```python
from build123d import *

# Parameters (mm, degrees)
SKETCH1_W           = 7
SKETCH1_H           = 6
BOSS_EXTRUDE1_DEPTH = 9
CUT_EXTRUDE1_DEPTH  = 2
CUT_EXTRUDE3_DEPTH  = 4
CUT_EXTRUDE4_DEPTH  = 7
SKETCH5_W           = 3
SKETCH5_H           = 2
CUT_EXTRUDE5_DEPTH  = 5
CUT_EXTRUDE8_DEPTH  = 4
CUT_EXTRUDE9_DEPTH  = 4
SKETCH11_W          = 2
SKETCH11_H          = 1
CUT_EXTRUDE12_DEPTH = 4
CUT_EXTRUDE13_DEPTH = 1
SKETCH13_W          = 1
SKETCH13_H          = 1
CUT_EXTRUDE14_DEPTH = 3


with BuildPart() as part:
    # Sketch1 → Boss-Extrude1 (new body)
    with BuildSketch(Plane.XY):
        Rectangle(SKETCH1_W, SKETCH1_H)
    extrude(amount=BOSS_EXTRUDE1_DEPTH)

    # Sketch2 → Cut-Extrude1 (cut)
    with BuildSketch(Plane(origin=(0, 3, 0), x_dir=(1, 0, 0), z_dir=(0, 1, 0))):
        Polygon((3.5, 0), (0.5, 0), (0.5, -3), align=None)
    extrude(amount=-CUT_EXTRUDE1_DEPTH, mode=Mode.SUBTRACT)

    # Sketch3 → Cut-Extrude3 (cut)
    with BuildSketch(Plane(origin=(0, 3, 0), x_dir=(1, 0, 0), z_dir=(0, 1, 0))):
        Polygon((3.5, 0), (0.5, -3), (0.5, -9), (3.5, -9), align=None)
    extrude(amount=-CUT_EXTRUDE3_DEPTH, mode=Mode.SUBTRACT)

    # Sketch4 → Cut-Extrude4 (cut, through all)
    with BuildSketch(Plane(origin=(0, 3, 0), x_dir=(1, 0, 0), z_dir=(0, 1, 0))):
        Polygon((3.5, 0), (1.5, -2), (1.5, -3), (0.5, -5), (0.5, -9), (3.5, -9), align=None)
    extrude(amount=-CUT_EXTRUDE4_DEPTH, mode=Mode.SUBTRACT)

    # Sketch5 → Cut-Extrude5 (cut, through all)
    with BuildSketch(Plane(origin=(0.5, 0, 0), x_dir=(0, 0, -1), z_dir=(1, 0, 0))):
        with Locations((-6.5, -2)):
            Rectangle(SKETCH5_W, SKETCH5_H)
    extrude(amount=-CUT_EXTRUDE5_DEPTH, mode=Mode.SUBTRACT)

    # Sketch7 → Cut-Extrude8 (cut)
    with BuildSketch(Plane(origin=(0, 3, 0), x_dir=(1, 0, 0), z_dir=(0, 1, 0))):
        Polygon((0.5, -3), (-0.5, -4), (-0.5, -9), (0.5, -9), align=None)
    extrude(amount=-CUT_EXTRUDE8_DEPTH, mode=Mode.SUBTRACT)

    # Sketch8 → Cut-Extrude9 (cut, through all)
    with BuildSketch(Plane(origin=(-0.5, 0, 0), x_dir=(0, 0, -1), z_dir=(1, 0, 0))):
        Polygon((-4, 3), (-5, 2), (-5, 1), (-7, 1), (-7, 3), align=None)
    extrude(amount=-CUT_EXTRUDE9_DEPTH, mode=Mode.SUBTRACT)

    # Sketch11 → Cut-Extrude12 (cut, through all)
    with BuildSketch(Plane(origin=(-0.5, 0, 0), x_dir=(0, 0, -1), z_dir=(1, 0, 0))):
        with Locations((-7, -0.5)):
            Rectangle(SKETCH11_W, SKETCH11_H)
    extrude(amount=-CUT_EXTRUDE12_DEPTH, mode=Mode.SUBTRACT)

    # Sketch12 → Cut-Extrude13 (cut)
    with BuildSketch(Plane(origin=(-0.5, 0, 0), x_dir=(0, 0, -1), z_dir=(1, 0, 0))):
        Polygon((-9, 3), (-7, 3), (-7, 1), (-6, 1), (-6, 0), (-8, 0), (-8, -1), (-9, -1), align=None)
    extrude(amount=-CUT_EXTRUDE13_DEPTH, mode=Mode.SUBTRACT)

    # Sketch13 → Cut-Extrude14 (cut, through all)
    with BuildSketch(Plane(origin=(0, -1, 0), x_dir=(1, 0, 0), z_dir=(0, 1, 0))):
        with Locations((0, -8.5)):
            Rectangle(SKETCH13_W, SKETCH13_H)
    extrude(amount=-CUT_EXTRUDE14_DEPTH, mode=Mode.SUBTRACT)


solid = part.part
```
Geometry: final body of the model. Coordinates: model frame, mm. A direction names the side the tool comes from. Coordinates: 2 decimals unless noted, no trailing zeros. Loops run counter-clockwise (first coordinate to the right, second up) from the corner with the lowest first, then second, coordinate; pieces in that order, holes last. Notation, with made-up numbers: M -28,3 L 0,3 A21 ccw 0,15 Z; hole C 37,64.5 d4. An arc over 180 degrees is marked long. Put each result on its own line as item: value.
(1) Cut plane A-A on y = -2. Return the cut outline in (x, z).
Answer sheet:
outline: M -3.5,0 L 3.5,0 L 1.5,2 L 1.5,3 L 0.5,5 L -3.5,5 Z; M -3.5,8 L -0.5,8 L -0.5,9 L -3.5,9 Z
(2) Cut plane C-C on x = -2.25. Return the cut outline in (y, z), then the cut area to 3 significant figures.
Answer sheet:
outline: M -3,0 L 3,0 L 3,4 L 2,5 L 1,5 L 1,7 L 3,7 L 3,9 L -3,9 L -3,8 L 0,8 L 0,6 L -1,6 L -1,5 L -3,5 Z
area: 41.5 mm^2
(3) Material intervals for probe 1 along Y at (x, z) = (0, 4); probe 2 along Z at (x, y) = (2, -0.25); probe 3 along X at (y, z) = (2, 8.75), sorted ascending.
Answer sheet:
probe 1: y = -3 to -1
probe 2: z = 0 to 1.5
probe 3: x = -3.5 to -1.5
(4) Access query for faces 1 (the face through (-2, 0, 7)), 2 (the face through (-1, -1, 8.5)), 3 (the face through (0.5, 2, 1)), 4 (the face through (-2, 2, 7)). Directions: +Z, -Z, +X, -X, +Y, -Y. A direction counts if a zero-diameter tool reaches every point of the face in a straight line with its end or side. Return the directions, or none.
Answer sheet:
face 1: +X, -X, -Y
face 2: +Z, +X, +Y
face 3: +Z, -Z, +X, +Y
face 4: +X, -X, +Y
(5) Draft query along Z for faces 5 (the face through (-2, 0, 9)), 6 (the face through (-2, -1, 5.5)), 7 (the face through (1.5, -2, 2.5)). Return one class per face: pulls with the +Z half, pulls with the -Z half, needs draft (parallel to the pull), parting line crosses it, or undercut.
Answer sheet:
face 5: pulls with the +Z half
face 6: undercut
face 7: needs draft
(6) First-contact query: pin 1 (1.6 mm diameter, centred on y = 2, z = 1, fed in from +X); pin 2 (0.5 mm diameter, centred on y = -2, z = 8.5, fed in from +X); pin 3 (0.5 mm diameter, centred on x = -2.5, z = 5.5, fed in from -Y). Flat tips, straight axial feed; report the tip coordinate or a pass-through.
Answer sheet:
pin 1: stops at x = 0.5
pin 2: stops at x = -0.5
pin 3: stops at y = -1
(7) Cut plane D-D on y = 0.75. Return the cut outline in (x, z).
Answer sheet:
outline: M -3.5,0 L 3.5,0 L -0.5,4 L -0.5,6 L -1.5,6 L -1.5,9 L -3.5,9 Z
(8) Cut plane B-B on z = 8.25. Return the cut outline in (x, y).
Answer sheet:
outline: M -3.5,-3 L -0.5,-3 L -0.5,-1 L -1.5,-1 L -1.5,3 L -3.5,3 Z
